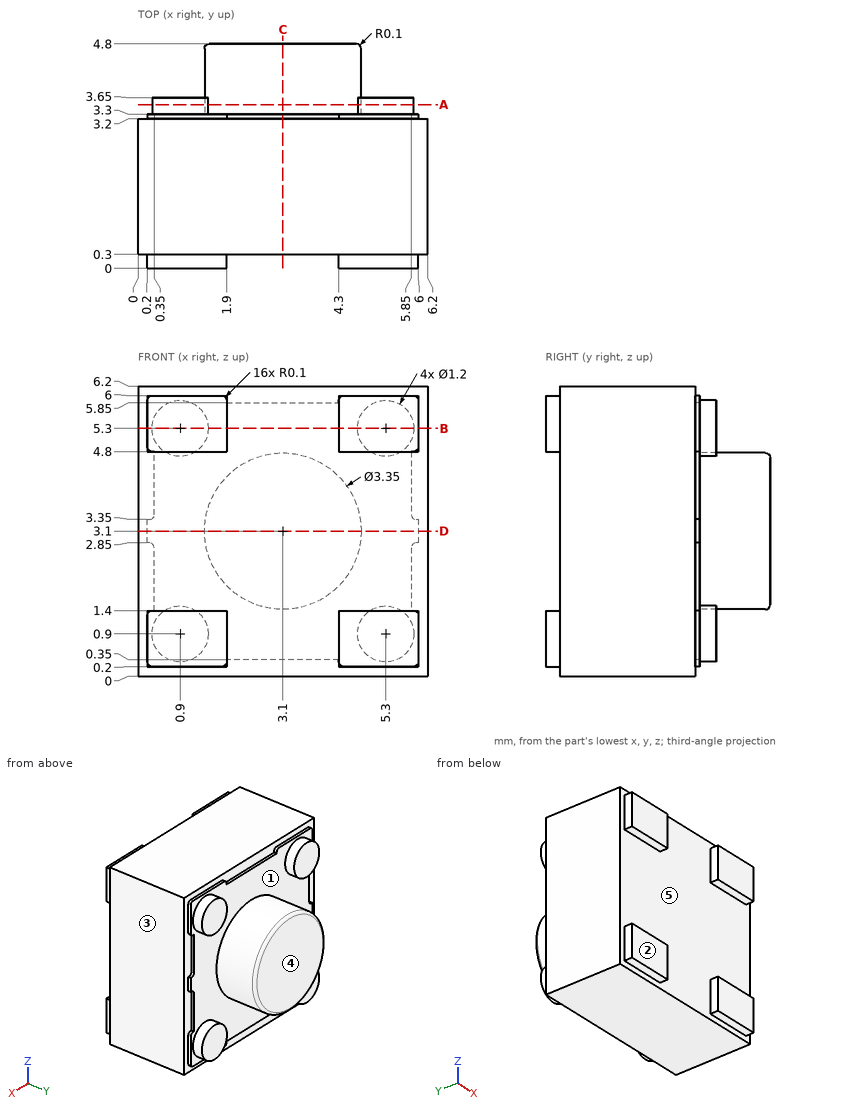
Answer from the drawing. Dimensions are ordinates in mm from the lowest x, y and z of the part. A direction names the side the tool comes from. Give positions to 0.01 mm unless a question says otherwise; leave off trailing zeros. Loops run counter-clockwise (first coordinate to the right, second up) from the corner with the lowest first, then second, coordinate; pieces in that order, holes last. Notation, with made-up numbers: (38, 32) -> (69, 32) arc R16 ccw to (69, 62) -> close; hole circle Ø11 at (-35.75, 78). An arc over 180 degrees is marked (long way). One line per question, with ' | ' between items. Start each with the question number.
1) For the marked faces 1 and 2, determine the directions among +Z, -Z, +X, -X, +Y, -Y from which every point of the face is accessible in a straight line to the end or side of a thin tool.
2) This flat-tipped pin is pushed along its axis until it touches: pin 1 (1.3 mm diameter, centred on x = 1, z = 5, fed in from +Y). Where does it stop, or does it pass through?
3) Section B-B, the plane z = 5.3 is taken. Determine the outline of the cut face in (x, y).
4) Straight lines are drawn through the part: L1, parallel to Y at x = 1.75, z = 0.75; L2, parallel to Y at x = 0.75, z = 2.25; L3, parallel to X at y = 3.4, z = 1.25. For each, find the intervals that lie inside material, in ascending order.
5) Section A-A, the plane y = 3.5 is taken. Determine the outline of the cut face in (x, z) (3 decimals), then the cut area to 3 significant figures.
6) Determine the mould class of the marked faces 3, 4 and 5 for opening direction X: +X half, -X half, draft (parallel to the pull), parting line (faces both ways), or undercut.
7) Section C-C, the plane x = 3.1 is taken. Determine the outline of the cut face in (y, z) (3 decimals).
8) Section D-D, the plane z = 3.1 is taken. Determine the outline of the cut face in (x, y) (3 decimals).
Resolved:
1) face 1: +Y | face 2: +Z, -Z, +X, -X, -Y
2) pin 1: y = 3.65
3) outline: (0, 0.3) -> (0.2, 0.3) -> (0.2, 0) -> (1.9, 0) -> (1.9, 0.3) -> (4.3, 0.3) -> (4.3, 0) -> (6, 0) -> (6, 0.3) -> (6.2, 0.3) -> (6.2, 3.2) -> (6, 3.2) -> (6, 3.3) -> (5.9, 3.3) -> (5.9, 3.65) -> (4.7, 3.65) -> (4.7, 3.3) -> (1.5, 3.3) -> (1.5, 3.65) -> (0.3, 3.65) -> (0.3, 3.3) -> (0.2, 3.3) -> (0.2, 3.2) -> (0, 3.2) -> close
4) L1: 0 to 3.3 | L2: 0.3 to 3.3 | L3: 0.41 to 1.39, 4.81 to 5.79
5) outline: circle Ø1.2 at (0.9, 0.9); circle Ø1.2 at (0.9, 5.3); circle Ø3.35 at (3.1, 3.1); circle Ø1.2 at (5.3, 0.9); circle Ø1.2 at (5.3, 5.3) | area: 13.3 mm2
6) face 3: +X half | face 4: draft | face 5: undercut
7) outline: (0.3, 0) -> (3.2, 0) -> (3.2, 0.35) -> (3.3, 0.35) -> (3.3, 1.425) -> (4.7, 1.425) arc R0.1 ccw to (4.8, 1.525) -> (4.8, 4.675) arc R0.1 ccw to (4.7, 4.775) -> (3.3, 4.775) -> (3.3, 5.85) -> (3.2, 5.85) -> (3.2, 6.2) -> (0.3, 6.2) -> close
8) outline: (0, 0.3) -> (6.2, 0.3) -> (6.2, 3.2) -> (6, 3.2) -> (6, 3.3) -> (4.775, 3.3) -> (4.775, 4.7) arc R0.1 ccw to (4.675, 4.8) -> (1.525, 4.8) arc R0.1 ccw to (1.425, 4.7) -> (1.425, 3.3) -> (0.2, 3.3) -> (0.2, 3.2) -> (0, 3.2) -> close
